Input: part model. Units: mm. Frame: model coordinates. Coordinates: 2 decimals unless noted, no trailing zeros. Write each loop counter-clockwise with the first axis right and the second up, starting at its lowest first coordinate (ties: lowest second). Pieces come first, ordered by that corner, then holes.
1) Pin query (flat end, axial travel): pin 1 Ø3 at (x, z) = (-2, -38.55) entering from +Y. Return the tip coordinate at first contact, or that it passes through.
2) Section query B-B (x = 16). Output: boundary loops of the cut face in (y, z), then the cut area to 3 significant figures.
3) Section query A-A (z = -38.55). Output: boundary loops of the cut face in (x, y).
4) Section query C-C (y = 1.8). State how many separate pieces and enclosed holes the cut face has, then the cut area to 3 significant figures.
5) Section query D-D (z = 50). Output: boundary loops of the cut face in (x, y).
6) Line query: L1, parallel to X at y = 1.1, z = 0; L2, parallel to X at y = 2.3, z = 38.55; L3, parallel to X at y = 2.6, z = -4.5. Output: solid intervals per line, ascending.
from build123d import *

# Parameters (mm, degrees)
SKETCH_1_R          = 2.5
SKETCH_1_R_2        = 2.45
SKETCH_1_R_3        = 1.85
SKETCH_1_W          = 48
SKETCH_1_H          = 40
EXTRUDE_1_DEPTH     = 3
CUT_EXTRUDE_1_REACH = 82.678
SKETCH_2_W          = 40
SKETCH_2_H          = 50


with BuildPart() as part:
    # 草图1 → 凸台-拉伸1 (new body)
    # profile 1 of 5: a face of its own
    with BuildSketch(Plane(origin=(0, 0, 0), x_dir=(1, 0, 0), z_dir=(0, 1, 0))):
        with BuildLine():
            Line((8, -30), (8, -70))
            Line((8, -70), (40, -70))
            Line((40, -70), (40, 60))
            Line((40, 60), (32.5, 60))
            ThreePointArc((32.5, 60), (28.232233047, 58.232233047), (30, 62.5))
            Line((30, 62.5), (30, 70))
            Line((30, 70), (8, 70))
            Line((8, 70), (8, 30))
            Line((8, 30), (-40, 30))
            Line((-40, 30), (-40, -30))
            Line((-40, -30), (8, -30))
        make_face()
        with Locations(Location((30, -60, 0), (0, 0, 270))):
            Circle(SKETCH_1_R, mode=Mode.SUBTRACT)
        with Locations(Location((30, 0, 0), (0, 0, 270))):
            Circle(SKETCH_1_R, mode=Mode.SUBTRACT)
    # profile 2 of 5: a face of its own
    with BuildSketch(Plane(origin=(0, 0, 0), x_dir=(1, 0, 0), z_dir=(0, 1, 0))):
        with BuildLine():
            Line((32.5, 60), (40, 60))
            Line((40, 60), (40, 70))
            Line((40, 70), (30, 70))
            Line((30, 70), (30, 62.5))
            ThreePointArc((30, 62.5), (31.767766953, 61.767766953), (32.5, 60))
        make_face()
    # profile 3 of 5: a face of its own
    with BuildSketch(Plane(origin=(0, 0, 0), x_dir=(1, 0, 0), z_dir=(0, 1, 0))):
        with BuildLine():
            Line((-40, 61.45), (-40, 30))
            Line((-40, 30), (8, 30))
            Line((8, 30), (8, 70))
            Line((8, 70), (-30, 70))
            Line((-30, 70), (-30, 63.3))
            ThreePointArc((-30, 63.3), (-28.691852455, 62.758147545), (-28.15, 61.45))
            ThreePointArc((-28.15, 61.45), (-30, 59.6), (-31.85, 61.45))
            Line((-31.85, 61.45), (-40, 61.45))
        make_face()
        with Locations(Location((-31.5, 50, 0), (0, 0, 270))):
            Circle(SKETCH_1_R_2, mode=Mode.SUBTRACT)
        with Locations(Location((-30, 38.55, 0), (0, 0, 270))):
            Circle(SKETCH_1_R_3, mode=Mode.SUBTRACT)
        with Locations(Location((-2, 38.55, 0), (0, 0, 270))):
            Circle(SKETCH_1_R_3, mode=Mode.SUBTRACT)
        with Locations(Location((-0.5, 50, 0), (0, 0, 270))):
            Circle(SKETCH_1_R_2, mode=Mode.SUBTRACT)
        with Locations(Location((-2, 61.45, 0), (0, 0, 270))):
            Circle(SKETCH_1_R_3, mode=Mode.SUBTRACT)
    # profile 4 of 5: a face of its own
    with BuildSketch(Plane(origin=(0, 0, 0), x_dir=(1, 0, 0), z_dir=(0, 1, 0))):
        with BuildLine():
            Line((-40, 70), (-40, 61.45))
            Line((-40, 61.45), (-31.85, 61.45))
            ThreePointArc((-31.85, 61.45), (-31.308147545, 62.758147545), (-30, 63.3))
            Line((-30, 63.3), (-30, 70))
            Line((-30, 70), (-40, 70))
        make_face()
    # profile 5 of 5: a face of its own
    with BuildSketch(Plane(origin=(0, 0, 0), x_dir=(1, 0, 0), z_dir=(0, 1, 0))):
        with Locations((-16, -50)):
            Rectangle(SKETCH_1_W, SKETCH_1_H)
        with Locations(Location((-30, -61.45, 0), (0, 0, 270))):
            Circle(SKETCH_1_R_3, mode=Mode.SUBTRACT)
        with Locations(Location((-31.5, -50, 0), (0, 0, 270))):
            Circle(SKETCH_1_R_2, mode=Mode.SUBTRACT)
        with Locations(Location((-30, -38.55, 0), (0, 0, 270))):
            Circle(SKETCH_1_R_3, mode=Mode.SUBTRACT)
        with Locations(Location((-2, -61.45, 0), (0, 0, 270))):
            Circle(SKETCH_1_R_3, mode=Mode.SUBTRACT)
        with Locations(Location((-0.5, -50, 0), (0, 0, 270))):
            Circle(SKETCH_1_R_2, mode=Mode.SUBTRACT)
        with Locations(Location((-2, -38.55, 0), (0, 0, 270))):
            Circle(SKETCH_1_R_3, mode=Mode.SUBTRACT)
    extrude(amount=EXTRUDE_1_DEPTH)

    # 草图2 → 切除-拉伸1 (cut, up to next)
    with BuildSketch(Plane(origin=(0, 3, 0), x_dir=(1, 0, 0), z_dir=(0, 1, 0)), mode=Mode.PRIVATE) as cut_extrude_1_sk1:
        Rectangle(SKETCH_2_W, SKETCH_2_H)
    cut_extrude_1_tool1 = extrude(cut_extrude_1_sk1.sketch, amount=-CUT_EXTRUDE_1_REACH, mode=Mode.PRIVATE) & part.part
    add(cut_extrude_1_tool1.solids().sort_by_distance((0, 3, 0))[0], mode=Mode.SUBTRACT)


solid = part.part
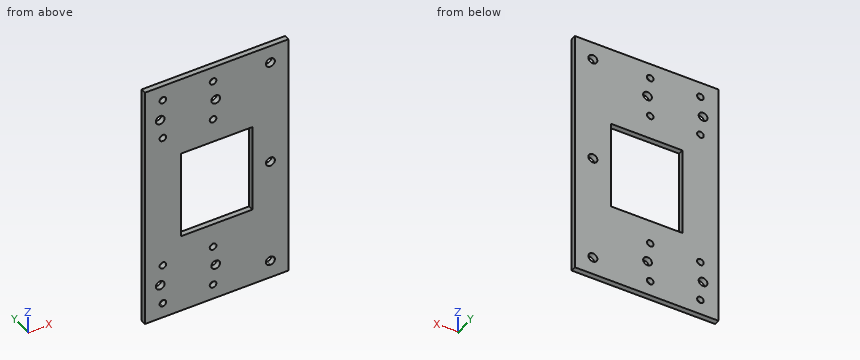
Answer:
1. pin 1: passes through
2. outline: (0, -70) - (3, -70) - (3, -25) - (0, -25) - close; (0, 25) - (3, 25) - (3, 70) - (0, 70) - close
2. area: 270 mm2
3. outline: (-40, 0) - (-31.85, 0) - (-31.85, 3) - (-40, 3) - close; (-28.15, 0) - (-3.85, 0) - (-3.85, 3) - (-28.15, 3) - close; (-0.15, 0) - (40, 0) - (40, 3) - (-0.15, 3) - close
4. separate pieces: 1
4. enclosed holes: 16
4. area: 8,980 mm2
5. outline: (-40, 0) - (-33.95, 0) - (-33.95, 3) - (-40, 3) - close; (-29.05, 0) - (-2.95, 0) - (-2.95, 3) - (-29.05, 3) - close; (1.95, 0) - (40, 0) - (40, 3) - (1.95, 3) - close
6. L1: x = -40 to -20, 20 to 27.5, 32.5 to 40
6. L2: x = -40 to -31.85, -28.15 to -3.85, -0.15 to 40
6. L3: x = -40 to -20, 20 to 40
